from build123d import *

# Parameters (mm, degrees)
SKETCH1_R         = 101.6
EXTRUDE1_DEPTH    = 22.352
SKETCH5_R         = 70
SKETCH5_R_2       = 67.46
EXTRUDE2_DEPTH    = 276.606
SKETCH6_R         = 4.2164
EXTRUDE3_DEPTH    = 332.694144905
CIRPATTERN1_COUNT = 20


with BuildPart() as part:
    # Sketch1 → Extrude1 (new body)
    with BuildSketch(Plane(origin=(0, 0, 0), x_dir=(1, 0, 0), z_dir=(0, 1, 0))):
        with Locations(Location((0, 0, 0), (0, 0, 270))):
            Circle(SKETCH1_R)
    extrude(amount=EXTRUDE1_DEPTH)

    # Sketch5 → Extrude2 (add)
    with BuildSketch(Plane.XZ):
        with Locations(Location((0, 0, 0), (0, 0, 90))):
            Circle(SKETCH5_R)
        with Locations(Location((0, 0, 0), (0, 0, 270))):
            Circle(SKETCH5_R_2, mode=Mode.SUBTRACT)
    extrude(amount=EXTRUDE2_DEPTH)

    # Sketch6 → Extrude3 (cut, through all)
    with BuildSketch(Plane(origin=(0, 22.352, 0), x_dir=(1, 0, 0), z_dir=(0, 1, 0))):
        with Locations(Location((0, 90.5256, 0), (0, 0, 270))):
            Circle(SKETCH6_R)
    extrude3 = extrude(amount=-EXTRUDE3_DEPTH, mode=Mode.SUBTRACT)

    # CirPattern1: Extrude3 ×20 about axis
    cirpattern1_axis = Axis((0, 0, 0), (0, 1, 0))
    for i in range(1, CIRPATTERN1_COUNT):
        add(extrude3.rotate(cirpattern1_axis, i * 360 / CIRPATTERN1_COUNT), mode=Mode.SUBTRACT)


solid = part.part
Work out the finished part from the listing and answer in its coordinate system (mm). A direction names the side the tool comes from. Give positions to 0.01 mm unless a question says otherwise; leave off trailing zeros. Order: outer loops, then holes, each group sorted by start corner. A loop starts at its lowest first (then second) coordinate and runs counter-clockwise, first axis right, second up. Notation, with made-up numbers: (85, -28) -> (101, -28) arc R31 cw to (101, 11) -> close; hole circle Ø5 at (11, -19). An arc over 180 degrees is marked (long way). One line per item, written item: value.
Item 1: Find section D-D, the plane x = -39. Give the vertices of the cut face in (y, z), plus the area to 3 significant figures.
Answer sheet:
outline: (-276.61, -58.13) -> (0, -58.13) -> (0, -93.82) -> (22.35, -93.82) -> (22.35, 93.82) -> (0, 93.82) -> (0, 58.13) -> (-276.61, 58.13) -> (-276.61, 55.04) -> (0, 55.04) -> (0, -55.04) -> (-276.61, -55.04) -> close
area: 5,900 mm²
Item 2: Find section A-A, the plane z = 0. Give the vertices of the cut face in (x, y).
Answer sheet:
outline: (-101.6, 0) -> (-94.74, 0) -> (-94.74, 22.35) -> (-101.6, 22.35) -> close; (-86.31, 0) -> (-70, 0) -> (-70, -276.61) -> (-67.46, -276.61) -> (-67.46, 0) -> (67.46, 0) -> (67.46, -276.61) -> (70, -276.61) -> (70, 0) -> (86.31, 0) -> (86.31, 22.35) -> (-86.31, 22.35) -> close; (94.74, 0) -> (101.6, 0) -> (101.6, 22.35) -> (94.74, 22.35) -> close
Item 3: Find section B-B, the plane x = 0. Give the vertices of the cut face in (y, z).
Answer sheet:
outline: (-276.61, -70) -> (0, -70) -> (0, -86.31) -> (22.35, -86.31) -> (22.35, 86.31) -> (0, 86.31) -> (0, 70) -> (-276.61, 70) -> (-276.61, 67.46) -> (0, 67.46) -> (0, -67.46) -> (-276.61, -67.46) -> close; (0, -101.6) -> (22.35, -101.6) -> (22.35, -94.74) -> (0, -94.74) -> close; (0, 94.74) -> (22.35, 94.74) -> (22.35, 101.6) -> (0, 101.6) -> close
Item 4: A tool of negligible diameter and unlimited length cuts with its end or side. For faces 3 (the flat face through (1, 0, -1)), 4 (the cylindrical face through (0.185, 11.332, -94.738)), from which of +Z, -Z, +X, -X, +Y, -Y can it reach the whole face along a straight path? Write none if from no direction.
Answer sheet:
face 3: -Y
face 4: +Y, -Y
Item 5: Determine the mould class of faces 1 (the cylindrical face through (-89.93, 11.33, 26.22)), 2 (the flat face through (-57, -276.606, -37)) for opening direction X: released by +X, released by -X, zero draft, split by the parting line, or undercut.
Answer sheet:
face 1: undercut
face 2: zero draft
Item 6: Find section C-C, the plane y = -58.5. Give the vertices of the cut face in (x, z), plus the area to 3 significant figures.
Answer sheet:
outline: circle Ø140 at (0, 0); hole circle Ø134.92 at (0, 0)
area: 1,100 mm²
Item 7: Flat-ended cylindrical pins translate along their axes: P1, Ø11, axis at x = -53.21, z = -73.24, coming from the +Y side; P2, Ø4, axis at y = -230, z = 40, coming from the +X side; P3, Ø3, axis at x = 49, y = -243.5, coming from the -Z side; P4, Ø1, axis at x = 33, z = -43, coming from the -Y side. Find the tip coordinate at first contact, or state that the pin passes through.
Answer sheet:
P1: y = 22.35
P2: x = 58.79
P3: z = -51.42
P4: y = 0
Item 8: Straight lines are drawn through the part: probe 1 along X at (y, z) = (-243, 1); probe 2 along Y at (x, z) = (81.5, -39); probe 3 along X at (y, z) = (-217, 49). For each, find the intervals that lie inside material, in ascending order.
Answer sheet:
probe 1: -69.99 to -67.45, 67.45 to 69.99
probe 2: 0 to 22.35
probe 3: -49.99 to -46.37, 46.37 to 49.99
